from build123d import *

# Parameters (mm, degrees)
SKETCH2_R           = 1.7
CUT_EXTRUDE1_DEPTH  = 25.532019892
SKETCH3_R           = 2.3
BOSS_EXTRUDE1_DEPTH = 4.6
CHAMFER1_SIZE       = 1
CHAMFER2_SIZE       = 1
CHAMFER2_SIZE2      = 1.732050808


with BuildPart() as part:
    # Sketch1 → Revolve1 (revolve)
    with BuildSketch(Plane.XY):
        Polygon((6, -0.9), (16.8, -0.9), (16.8, -0.5), (17.3, 0), (16.8, 0.5), (16.8, 0.9), (6, 0.9), align=None)
    revolve(axis=Axis((0, -175.207382849, 0), (0, 1, 0)))

    # Sketch2 → Cut-Extrude1 (cut, through all)
    with BuildSketch(Plane(origin=(0, 0.9, 0), x_dir=(1, 0, 0), z_dir=(0, 1, 0))):
        with Locations(Location((0, 9.385, 0), (0, 0, 180))):
            Circle(SKETCH2_R)
        with Locations(Location((8.127648415, 4.6925, 0), (0, 0, 180))):
            Circle(SKETCH2_R)
        with Locations(Location((8.127648415, -4.6925, 0), (0, 0, 180))):
            Circle(SKETCH2_R)
        with Locations(Location((0, -9.385, 0), (0, 0, 180))):
            Circle(SKETCH2_R)
        with Locations(Location((-8.127648415, -4.6925, 0), (0, 0, 180))):
            Circle(SKETCH2_R)
        with Locations(Location((-8.127648415, 4.6925, 0), (0, 0, 180))):
            Circle(SKETCH2_R)
    extrude(amount=-CUT_EXTRUDE1_DEPTH, mode=Mode.SUBTRACT)

    # Sketch3 → Boss-Extrude1 (add)
    with BuildSketch(Plane.XZ.offset(0.9)):
        with Locations((6.75, 11.691342951)):
            Circle(SKETCH3_R)
        with Locations((-6.75, -11.691342951)):
            Circle(SKETCH3_R)
    extrude(amount=BOSS_EXTRUDE1_DEPTH)

    # Chamfer1
    chamfer1_edges = [part.edges().sort_by_distance(p)[0] for p in [
        (4.45, -5.5, 11.691342951),
        (-9.05, -5.5, -11.691342951),
    ]]
    chamfer(chamfer1_edges, length=CHAMFER1_SIZE)

    # Chamfer2
    chamfer2_edges = [part.edges().sort_by_distance(p)[0] for p in [
        (-6, -0.9, 0),
    ]]
    chamfer2_side = [part.faces().sort_by_distance(p)[0] for p in [
        (-16.324824243, -0.9, 0),
    ]]
    chamfer(chamfer2_edges, length=CHAMFER2_SIZE, length2=CHAMFER2_SIZE2, reference=chamfer2_side[0])


solid = part.part
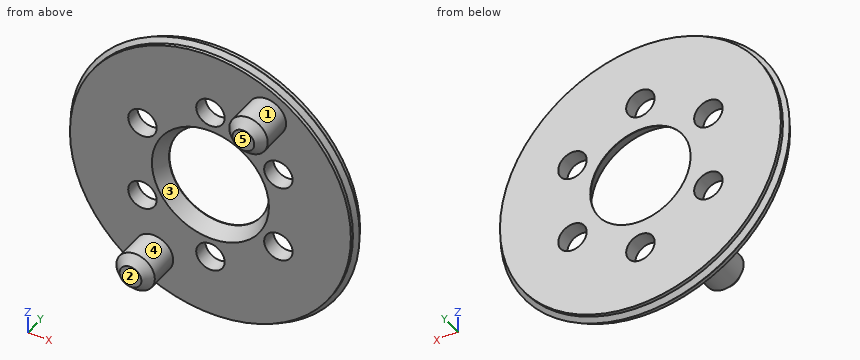
The listing builds one solid part. Answer for the finished solid, in the listing's coordinates (mm). Face numbers are marked on the shaded views. A direction names the side the tool comes from. Round coordinates to 2 decimals unless told otherwise and drop trailing zeros. Order: outer loops, then holes, each group sorted by start corner. A loop starts at its lowest first (then second) coordinate and runs counter-clockwise, first axis right, second up. Notation, with made-up numbers: (-28.75, -6) -> (26.25, -6) arc R16 cw to (26.25, 23) -> close; hole circle Ø1 at (0.25, 1.5). An arc over 180 degrees is marked (long way). Put each result on its own line as item: value.
Q1. Each of these flat-tipped pins is pushed along its axis until it touches: P1, Ø4, axis at x = -8.13, z = -4.69, coming from the -Y side; P2, Ø3, axis at y = -2, z = -11, coming from the +X side; P3, Ø2.5, axis at x = 8.13, z = 4.69, coming from the -Y side; P4, Ø1.5, axis at y = -0.5, z = 12, coming from the +X side. Where does it stop, or does it pass through?
Results list:
P1: y = -0.9
P2: x = 13.51
P3: through
P4: x = 12.98
Q2. Section C-C, the plane y = -3.25 is taken. Write down the section's boundary in (x, z), and give its area (3 significant figures).
Results list:
outline: circle Ø4.6 at (-6.75, -11.69); circle Ø4.6 at (6.75, 11.69)
area: 33.2 mm^2
Q3. Section B-B, the plane z = 0 is taken. Write down the section's boundary in (x, y), and give its area (3 significant figures).
Results list:
outline: (-17.3, 0) -> (-16.8, -0.5) -> (-16.8, -0.9) -> (-7, -0.9) -> (-6, 0.83) -> (-6, 0.9) -> (-16.8, 0.9) -> (-16.8, 0.5) -> close; (6, 0.83) -> (7, -0.9) -> (16.8, -0.9) -> (16.8, -0.5) -> (17.3, 0) -> (16.8, 0.5) -> (16.8, 0.9) -> (6, 0.9) -> close
area: 37.6 mm^2
Q4. Consider line 1 along X through (y, z) = (-0.75, 4); line 2 along Z through (x, y) = (-9, -0.5); line 3 along Y through (x, z) = (7, -7). Determine where each line is inside the solid, lowest interval first.
Results list:
line 1: -16.32 to -9.68, -6.58 to -5.64, 5.64 to 6.58, 9.68 to 16.32
line 2: -14.19 to -6.15, -3.23 to 3.23, 6.15 to 14.19
line 3: -0.9 to 0.9
Q5. Section A-A, the plane x = 0 is taken. Write down the section's boundary in (y, z) (3 decimals), and give its area (3 significant figures).
Results list:
outline: (-0.9, -16.8) -> (-0.5, -16.8) -> (0, -17.3) -> (0.5, -16.8) -> (0.9, -16.8) -> (0.9, -11.085) -> (-0.9, -11.085) -> close; (-0.9, -7.685) -> (0.9, -7.685) -> (0.9, -6) -> (0.832, -6) -> (-0.9, -7) -> close; (-0.9, 7) -> (0.832, 6) -> (0.9, 6) -> (0.9, 7.685) -> (-0.9, 7.685) -> close; (-0.9, 11.085) -> (0.9, 11.085) -> (0.9, 16.8) -> (0.5, 16.8) -> (0, 17.3) -> (-0.5, 16.8) -> (-0.9, 16.8) -> close
area: 25.4 mm^2
Q6. Determine the mould class of the marked faces 1, 2 and 3 for opening direction X: pulls with the +X half, pulls with the -X half, needs draft (parallel to the pull), parting line crosses it, or undercut.
Results list:
face 1: parting line crosses it
face 2: needs draft
face 3: undercut
Q7. Which of the six approach directions +Z, -Z, +X, -X, +Y, -Y give full straight-line access (tool end or side, diameter ignored) to the marked faces 4 and 5?
Results list:
face 4: -Y
face 5: +Z, -Z, +X, -X, -Y
